from build123d import *

# Parameters (mm, degrees)
F1_DEPTH = 12
F2_DEPTH = 25


# Not quite as in the source:
# - ends of sketch curves that miss each other by under 0.0002 mm in the source are joined


with BuildPart() as f1:
    # F0 (on Top) → F1 (new body)
    with BuildSketch(Plane.XY):
        with BuildLine():
            Line((-45.2079510631, 38.1848650801), (-50.0674114416, 38.1848649627))
            ThreePointArc((-50.0674114416, 38.1848649627), (-51.7515474497, 34.119000832), (-55.8174114415, 32.4348648238))
            Line((-55.8174114415, 32.4348648238), (-55.8174114414, 29.083605512))
            Line((-55.8174114414, 29.083605512), (-44.5532578407, 15.1687110318))
            ThreePointArc((-44.5532578407, 15.1687110318), (-42.1350647352, 24.8048651036), (-35.4555304308, 32.1592477879))
            Line((-35.4555304308, 32.1592477879), (-45.2079510631, 38.1848650801))
        make_face()
        with BuildLine():
            Line((-50.0674114416, 38.1848649627), (-52.4674114416, 38.1848649047))
            ThreePointArc((-52.4674114416, 38.1848649047), (-53.4486037246, 35.8160571069), (-55.8174114415, 34.8348648238))
            Line((-55.8174114415, 34.8348648238), (-55.8174114415, 32.4348648238))
            ThreePointArc((-55.8174114415, 32.4348648238), (-51.7515474497, 34.119000832), (-50.0674114416, 38.1848649627))
        make_face()
        with BuildLine():
            Line((-55.8174114414, 29.083605512), (-55.8174114415, 32.4348648238))
            ThreePointArc((-55.8174114415, 32.4348648238), (-58.0556968865, 32.8883963526), (-59.9408925855, 34.1774462962))
            Line((-59.9408925855, 34.1774462962), (-55.8174114414, 29.083605512))
        make_face()
        with BuildLine():
            Line((-55.8174114415, 32.4348648238), (-55.8174114415, 34.8348648238))
            ThreePointArc((-55.8174114415, 34.8348648238), (-57.1214560051, 35.0990962362), (-58.2197874124, 35.8501079425))
            Line((-58.2197874124, 35.8501079425), (-59.9408925855, 34.1774462962))
            ThreePointArc((-59.9408925855, 34.1774462962), (-58.0556968865, 32.8883963526), (-55.8174114415, 32.4348648238))
        make_face()
        with BuildLine():
            ThreePointArc((-58.2197874124, 35.8501079425), (-58.1521683229, 40.5872407946), (-53.4150354708, 40.5196217052))
            Line((-53.4150354708, 40.5196217052), (-51.6939302977, 42.1922833515))
            ThreePointArc((-51.6939302977, 42.1922833515), (-59.8248299692, 42.3083459677), (-59.9408925855, 34.1774462962))
            Line((-59.9408925855, 34.1774462962), (-58.2197874124, 35.8501079425))
        make_face()
        with BuildLine():
            ThreePointArc((-53.4150354708, 40.5196217052), (-52.7133447942, 39.4447339634), (-52.4674114416, 38.1848648238))
            Line((-52.4674114416, 38.1848648238), (-50.0674114416, 38.1848649627))
            ThreePointArc((-50.0674114416, 38.1848649627), (-50.4895358529, 40.3473267799), (-51.6939302977, 42.1922833515))
            Line((-51.6939302977, 42.1922833515), (-53.4150354708, 40.5196217052))
        make_face()
        with BuildLine():
            ThreePointArc((-51.6939302977, 42.1922833515), (-50.4895358529, 40.3473267799), (-50.0674114416, 38.1848648238))
            Line((-50.0674114416, 38.1848648238), (-45.2079510631, 38.1848650801))
            Line((-45.2079510631, 38.1848650801), (-51.6939302977, 42.1922833515))
        make_face()
        with BuildLine():
            ThreePointArc((-24.1338443596, 35.5853722206), (-30.0482104313, 34.7100811604), (-35.4555304308, 32.1592477879))
            ThreePointArc((-35.4555304308, 32.1592477879), (-42.1350647352, 24.8048651036), (-44.5532578407, 15.1687110318))
            Line((-44.5532578407, 15.1687110318), (-42.6338443592, 15.1659585535))
            Line((-42.6338443592, 15.1659585535), (-39.8838443592, 15.1659585535))
            ThreePointArc((-39.8838443592, 15.1659585535), (-35.270776163, 26.3028903571), (-24.1338443595, 30.9159585535))
            Line((-24.1338443595, 30.9159585535), (-24.1338443596, 35.5853722206))
        make_face()
        with BuildLine():
            ThreePointArc((-3.7144306922, 15.1659585535), (-9.6951384875, 29.6046644255), (-24.1338443596, 35.5853722206))
            Line((-24.1338443596, 35.5853722206), (-24.1338443595, 30.9159585535))
            ThreePointArc((-24.1338443595, 30.9159585535), (-12.9969125556, 26.3028903573), (-8.3838443592, 15.1659585535))
            Line((-8.3838443592, 15.1659585535), (-5.6338443592, 15.1659585535))
            Line((-5.6338443592, 15.1659585535), (-3.7144306922, 15.1659585535))
        make_face()
        with BuildLine():
            Line((-42.6338443592, 15.1659585535), (-44.5532578407, 15.1687110318))
            ThreePointArc((-44.5532578407, 15.1687110318), (-42.7914410163, 6.8685769492), (-37.807970261, 0.0011725238))
            Line((-37.807970261, 0.0011725238), (-38.0284454354, 0.643162408))
            Line((-38.0284454354, 0.643162408), (-35.5289696075, 0.5919707473))
            Line((-35.5289696075, 0.5919707473), (-42.6338443592, 15.1659585535))
        make_face()
        Polygon((-38.0284454354, 0.643162408), (-37.807970261, 0.0011725238), (-35.1236572441, -7.8151351762), (-32.6315665225, -7.8151351762), (-35.5289696075, 0.5919707473), align=None)
        Polygon((-32.6315665225, -7.8151351762), (-35.1236572441, -7.8151351762), (-32.8838443592, -14.3371266833), (-30.3838443592, -14.3371266833), align=None)
        Polygon((-13.136122196, -7.8151351762), (-15.636122196, -7.8151351762), (-17.8838443592, -14.3371266833), (-15.3838443592, -14.3371266833), align=None)
        Polygon((-10.2387191109, 0.5919707473), (-12.7387191109, 0.5919707473), (-15.636122196, -7.8151351762), (-13.136122196, -7.8151351762), (-10.4427343672, 0), align=None)
        with BuildLine():
            Line((7.5497227229, 2.079326472), (-3.7144306922, 15.1659585535))
            Line((-3.7144306922, 15.1659585535), (-5.6338443592, 15.1659585535))
            Line((-5.6338443592, 15.1659585535), (-12.7387191109, 0.5919707473))
            Line((-12.7387191109, 0.5919707473), (-10.2387191109, 0.5919707473))
            Line((-10.2387191109, 0.5919707473), (-10.4427343672, 0))
            Line((-10.4427343672, 0), (-0.3331204375, -7.8151351762))
            Line((-0.3331204375, -7.8151351762), (1.9170354556, -7.8151351762))
            ThreePointArc((1.9170354556, -7.8151351762), (3.0939956275, -3.0251503303), (7.549722723, -0.909568585))
            Line((7.549722723, -0.909568585), (7.5497227229, 2.079326472))
        make_face()
        with BuildLine():
            ThreePointArc((13.2997227231, -6.659568585), (12.7982725871, -4.3111171112), (11.3813838275, -2.3722765282))
            Line((11.3813838275, -2.3722765282), (9.7820818013, -4.1617549519))
            ThreePointArc((9.7820818013, -4.1617549519), (10.6075735134, -5.2913403351), (10.8997227231, -6.659568585))
            ThreePointArc((10.8997227231, -6.659568585), (8.917950973, -9.7174193754), (5.3173636448, -9.1573822181))
            Line((5.3173636448, -9.1573822181), (3.7180616186, -10.9468606418))
            ThreePointArc((3.7180616186, -10.9468606418), (9.8981741968, -11.908118449), (13.2997227231, -6.659568585))
        make_face()
        with BuildLine():
            ThreePointArc((11.3813838275, -2.3722765282), (9.6004019609, -1.2876774223), (7.549722723, -0.909568585))
            Line((7.549722723, -0.909568585), (7.549722723, -3.309568585))
            ThreePointArc((7.549722723, -3.309568585), (8.744466279, -3.5298580815), (9.7820818013, -4.1617549519))
            Line((9.7820818013, -4.1617549519), (11.3813838275, -2.3722765282))
        make_face()
        with BuildLine():
            Line((7.549722723, -3.309568585), (7.549722723, -0.909568585))
            ThreePointArc((7.549722723, -0.909568585), (3.0939956275, -3.0251503303), (1.9170354556, -7.8151351762))
            ThreePointArc((1.9170354556, -7.8151351762), (2.5652068364, -9.5261172721), (3.7180616186, -10.9468606418))
            Line((3.7180616186, -10.9468606418), (5.3173636448, -9.1573822181))
            ThreePointArc((5.3173636448, -9.1573822181), (4.4200122196, -5.464825029), (7.549722723, -3.309568585))
        make_face()
        with BuildLine():
            ThreePointArc((3.7180616186, -10.9468606418), (2.5652068364, -9.5261172721), (1.9170354556, -7.8151351762))
            Line((1.9170354556, -7.8151351762), (-0.3331204375, -7.8151351762))
            Line((-0.3331204375, -7.8151351762), (3.7180616186, -10.9468606418))
        make_face()
        with BuildLine():
            Line((11.3813838275, -2.3722765282), (7.5497227229, 2.079326472))
            Line((7.5497227229, 2.079326472), (7.549722723, -0.909568585))
            ThreePointArc((7.549722723, -0.909568585), (9.6004019609, -1.2876774223), (11.3813838275, -2.3722765282))
        make_face()
    extrude(amount=F1_DEPTH)

    # F0 (on Top) → F2 (join)
    with BuildSketch(Plane.XY):
        Polygon((-38.0284454354, 0.643162408), (-37.807970261, 0.0011725238), (-35.1236572441, -7.8151351762), (-32.6315665225, -7.8151351762), (-35.5289696075, 0.5919707473), align=None)
        Polygon((-32.6315665225, -7.8151351762), (-35.1236572441, -7.8151351762), (-32.8838443592, -14.3371266833), (-30.3838443592, -14.3371266833), align=None)
        Polygon((-13.136122196, -7.8151351762), (-15.636122196, -7.8151351762), (-17.8838443592, -14.3371266833), (-15.3838443592, -14.3371266833), align=None)
        Polygon((-10.2387191109, 0.5919707473), (-12.7387191109, 0.5919707473), (-15.636122196, -7.8151351762), (-13.136122196, -7.8151351762), (-10.4427343672, 0), align=None)
    extrude(amount=F2_DEPTH)


solid = f1.part
Check sheet for the modelled part. Datum: model origin and axes. Units: mm. A direction names the side the tool comes from. Coordinates: 2 decimals unless noted, no trailing zeros. Loops run counter-clockwise (first coordinate to the right, second up) from the corner with the lowest first, then second, coordinate; pieces in that order, holes last. Notation, with made-up numbers: (49.5, -26.5) -> (58.5, -26.5) arc R20 cw to (58.5, 0.5) -> close; hole circle Ø4 at (29, -26.5). An arc over 180 degrees is marked (long way). Write item = value, one per line. Start each with the question number.
1. Depth check by flat-ended pin: P1, Ø10, axis at y = 19.5, z = 15.5, coming from the +X side; P2, Ø10, axis at x = -47.5, y = 34.5, coming from the +Z side; P3, Ø2, axis at x = -7.5, z = 5.5, coming from the -Y side; P4, Ø1, axis at x = -41.5, y = 26, coming from the -Z side. Enter the tip coordinate at first touch or a pass-through.
2. Material ranges on line 1 (X direction, y = -2, z = 4.5); line 2 (X direction, y = -7, z = 3); line 3 (Z direction, x = -45.5, y = 18), recorded low to high.
3. Section check C-C on x = -21. Record the cut outline in (y, z).
4. Section check B-B on z = 5.75. Record the cut outline in (x, y).
5. Tool access check on faces 1 (the flat face through (-32, -14.337, 12)), 2 (the flat face through (-39.032, 7.777, 5.916)). Record the directions out of +Z, -Z, +X, -X, +Y, -Y that give a thin tool (end or side, any length) a straight path to the whole face; none if there is none.
6. Section check A-A on z = 22.75. Record the cut outline in (x, y).
7. Draft check along Y on faces 3 (the cylindrical face through (-59.73, 42.4, 5.92)), 4 (the flat face through (-9.137, 7.981, 5.916)), 5 (the flat face through (-30, 30, 0)). Enter one of: released by +Y, released by -Y, zero draft, split by the parting line, or undercut.
Responses:
q1.P1 = -3.73
q1.P2 = 12
q1.P3 = -3.05
q1.P4 = 0
q2.line_1 = -37.12 to -34.64, -13.63 to -11.13, -7.86 to 11.06
q2.line_2 = -35.4 to -32.91, -15.36 to -12.86, -1.39 to 4.22, 10.88 to 13.29
q2.line_3 = 0 to 12
q3.outline = (30.6, 0) -> (35.34, 0) -> (35.34, 12) -> (30.6, 12) -> close
q4.outline = (-59.94, 34.18) -> (-44.55, 15.17) arc R20.42 ccw to (-37.81, 0) -> (-32.88, -14.34) -> (-30.38, -14.34) -> (-35.53, 0.59) -> (-42.63, 15.17) -> (-39.88, 15.17) arc R15.75 cw to (-8.38, 15.17) -> (-5.63, 15.17) -> (-12.74, 0.59) -> (-17.88, -14.34) -> (-15.38, -14.34) -> (-10.44, 0) -> (3.72, -10.95) arc R5.75 ccw to (11.38, -2.37) -> (-3.71, 15.17) arc R20.42 ccw to (-35.46, 32.16) -> (-51.69, 42.19) arc R5.75 ccw to start; hole circle Ø6.7 at (-55.82, 38.18); hole circle Ø6.7 at (7.55, -6.66)
q5.face_1 = +Z, -Z, +X, -X, -Y
q5.face_2 = +Z, -Z
q6.outline = (-38.03, 0.64) -> (-32.88, -14.34) -> (-30.38, -14.34) -> (-35.53, 0.59) -> close; (-17.88, -14.34) -> (-15.38, -14.34) -> (-10.24, 0.59) -> (-12.74, 0.59) -> close
q7.face_3 = split by the parting line
q7.face_4 = undercut
q7.face_5 = zero draft
